from build123d import *

# Parameters (mm, degrees)
BOSS_EXTRUDE2_DEPTH      = 25.4
BOSS_EXTRUDE2_DEPTH_BACK = 25.4
SKETCH5_W                = 55.996028866
SKETCH5_H                = 43.041519522
CUT_EXTRUDE2_DEPTH       = 71.12
CUT_EXTRUDE4_REACH       = 104.359
SKETCH8_W                = 20.066
SKETCH8_H                = 41.148


with BuildPart() as part:
    # Sketch3 → Boss-Extrude2 (new, two sides: drawn at the far end of the back side and taken through both)
    with BuildSketch(Plane.XY.offset(-BOSS_EXTRUDE2_DEPTH_BACK)):
        with BuildLine():
            Line((-31.917133282, 0), (18.882866718, 0))
            Line((18.882866718, 0), (18.882866718, 50.8))
            Line((18.882866718, 50.8), (16.643514063, 63.5))
            ThreePointArc((16.643514063, 63.5), (-6.517133282, 82.934090645), (-29.677780627, 63.5))
            Line((-29.677780627, 63.5), (-31.917133282, 50.8))
            Line((-31.917133282, 50.8), (-31.917133282, 0))
        make_face()
    extrude(amount=BOSS_EXTRUDE2_DEPTH + BOSS_EXTRUDE2_DEPTH_BACK)

    # Sketch5 → Cut-Extrude2 (cut)
    with BuildSketch(Plane(origin=(0, 82.934090645, 0), x_dir=(1, 0, 0), z_dir=(0, 1, 0))):
        with Locations((-7.030712477, -4.838222216)):
            Rectangle(SKETCH5_W, SKETCH5_H)
    extrude(amount=-CUT_EXTRUDE2_DEPTH, mode=Mode.SUBTRACT)

    # Sketch8 → Cut-Extrude4 (cut, up to next)
    with BuildSketch(Plane.XY.offset(25.4), mode=Mode.PRIVATE) as cut_extrude4_sk1:
        with Locations((-6.517133282, 43.625792805)):
            Rectangle(SKETCH8_W, SKETCH8_H)
    cut_extrude4_tool1 = extrude(cut_extrude4_sk1.sketch, amount=-CUT_EXTRUDE4_REACH, mode=Mode.PRIVATE) & part.part
    add(cut_extrude4_tool1.solids().sort_by_distance((-6.517133, 43.625793, 25.4))[0], mode=Mode.SUBTRACT)


solid = part.part
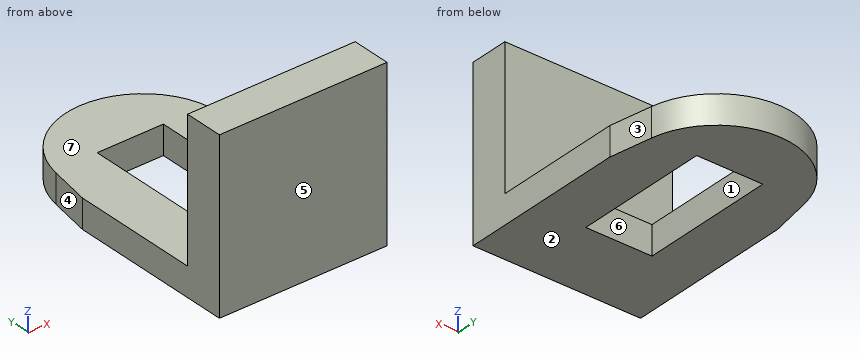
Here's how the part is built. I have some questions about the finished solid (model axes, mm). Face numbers are marked on the shaded views. A direction names the side the tool comes from. Coordinates: 2 decimals unless noted, no trailing zeros. Order: outer loops, then holes, each group sorted by start corner. A loop starts at its lowest first (then second) coordinate and runs counter-clockwise, first axis right, second up.
Item 1: For the marked faces 5, 6 and 7, which set-ups out of +Z, -Z, +X, -X, +Y, -Y let a thin tool reach every point of the face, with its end or its side?
Result sheet:
face 5: +Z, -Z, +X, -X, -Y
face 6: +Z, -Z
face 7: +Z, +X, -X, +Y
Item 2: I need wall thicknesses on line 1 (Y direction, x = -30, z = -1); line 2 (Z direction, x = -10.5, y = 75.5); line 3 (X direction, y = 56.5, z = -22.5). Which ranges of each line are inside material? Lowest first, please.
Result sheet:
line 1: y = 0 to 11.81
line 2: z = -25.4 to -16.68
line 3: x = -30.91 to -16.55, 3.52 to 17.88
Item 3: If we section it at C-C on z = 8: List the corners of the cut face in (x, y) for me, plus the area to 3 significant figures.
Result sheet:
outline: (-31.92, 0) - (18.88, 0) - (18.88, 11.81) - (-31.92, 11.81) - close
area: 600 mm2
Item 4: If we section it at B-B on x = -15.5: List the corners of the cut face in (y, z) for me, plus the area to 3 significant figures.
Result sheet:
outline: (0, -25.4) - (23.05, -25.4) - (23.05, -16.68) - (11.81, -16.68) - (11.81, 25.4) - (0, 25.4) - close; (64.2, -25.4) - (81.15, -25.4) - (81.15, -16.68) - (64.2, -16.68) - close
area: 846 mm2
Item 5: If we section it at D-D on y = 15: List the corners of the cut face in (x, z) for me.
Result sheet:
outline: (-31.92, -25.4) - (18.88, -25.4) - (18.88, -16.68) - (-31.92, -16.68) - close
Item 6: If we section it at A-A on y = 27: List the corners of the cut face in (x, z) for me, plus the area to 3 significant figures.
Result sheet:
outline: (-31.92, -25.4) - (-16.55, -25.4) - (-16.55, -16.68) - (-31.92, -16.68) - close; (3.52, -25.4) - (18.88, -25.4) - (18.88, -16.68) - (3.52, -16.68) - close
area: 268 mm2
Item 7: If we mould it in two halves opening along X, with no side actions, what happens to the marked faces 1, 2, 3 and 4? For each: +X half, -X half, draft (parallel to the pull), parting line (faces both ways), or undercut.
Result sheet:
face 1: undercut
face 2: draft
face 3: +X half
face 4: -X half
Item 8: For P1, Ø1.5, axis at x = 12, z = -14.5, coming from the -Y side; P2, Ø21, axis at x = 4, z = 2, coming from the +Y side; P3, Ø6, axis at x = 7, y = 65.5, coming from the +Z side; P4, Ø4.5, axis at x = -11.5, z = -19.5, coming from the +Y side, each with a flat end and sliding along its axis, tell me the tip position at first contact or that it passes through.
Result sheet:
P1: stops at y = 0
P2: stops at y = 11.81
P3: stops at z = -16.68
P4: stops at y = 82.77
